```python
from build123d import *

# Parameters (mm, degrees)
F1_DEPTH = 2.159


with BuildPart() as f1:
    # F0 (on Top) → F1 (new body)
    with BuildSketch(Plane.XY):
        with BuildLine():
            add(Edge.make_bspline(
                [(32.7343828976, 20.32), (49.2011681199, 17.9275516421), (66.9959262013, 9.6941580996), (76.2, -8.8973781094)],
                knots=[0, 0, 0, 0, 52.3728465302, 52.3728465302, 52.3728465302, 52.3728465302], degree=3))
            Line((32.7343828976, 20.32), (-76.2, 20.32))
            Line((-76.2, 20.32), (-88.9, 20.32))
            Line((-88.9, 20.32), (-88.9, 14.9225))
            Line((-88.9, 14.9225), (-114.3, 14.9225))
            Line((-114.3, 14.9225), (-114.3, 7.3025))
            Line((-114.3, 7.3025), (-88.9, 7.3025))
            Line((-88.9, 7.3025), (-88.9, 1.905))
            ThreePointArc((-88.9, 1.905), (-79.9197438789, -1.8147438789), (-76.2, -10.795))
            Line((-76.2, -10.795), (-76.2, -20.32))
            add(Edge.make_bspline(
                [(-76.2, -20.32), (-27.4205083204, -20.32), (18.5684725391, -19.3262068454), (60.0895812138, -13.8769824012), (76.2, -8.8973781094)],
                knots=[0, 0, 0, 0, 0.5808971053, 1, 1, 1, 1], degree=3))
        make_face()
    extrude(amount=F1_DEPTH)


solid = f1.part
```
Input: part model. Units: mm. Frame: model coordinates. Give positions to 0.01 mm unless a question says otherwise; leave off trailing zeros. Order: outer loops, then holes, each group sorted by start corner. A loop starts at its lowest first (then second) coordinate and runs counter-clockwise, first axis right, second up. Notation, with made-up numbers: M 12.25,50 L 46.25,50 A27 ccw 46.25,85 Z; hole C 10.25,-6.5 d8. An arc over 180 degrees is marked long. Return JSON: item names as keys, results as strings.
1) Line query: L1, parallel to Y at x = -88, z = 1.7; L2, parallel to Y at x = -35.5, z = 1.25; L3, parallel to X at y = -2, z = 1.3. Output: solid intervals per line, ascending. Write a range as [from, to].
Taken from the geometry:
{"L1": "y = [1.87, 20.32]", "L2": "y = [-20.11, 20.32]", "L3": "x = [-79.74, 72.08]"}
2) Contact query for flat-ended pins moving along their axis: pin 1 (0.6 mm diameter, centred on y = 18, z = 1.5, fed in from -X); pin 2 (1 mm diameter, centred on x = -40.5, z = 0.5, fed in from -Y); pin 3 (1.1 mm diameter, centred on y = -14.5, z = 0.5, fed in from -X). Output: stop coordinate, or through.
Taken from the geometry:
{"pin 1": "stops at x = -88.9", "pin 2": "stops at y = -20.17", "pin 3": "stops at x = -76.2"}
3) Section query A-A on x = -80. Output: boundary loops of the cut face in (y, z), and give its area (3 significant figures).
Taken from the geometry:
{"outline": "M -1.74,0 L 20.32,0 L 20.32,2.16 L -1.74,2.16 Z", "area": "47.6 mm2"}
